```python
from build123d import *

# Parameters (mm, degrees)
SKETCH_1_W          = 35
SKETCH_1_H          = 25
EXTRUDE_1_DEPTH     = 10
SKETCH_1_4_W        = 10
SKETCH_1_4_H        = 25
EXTRUDE_2_DEPTH     = 15
SKETCH_2_W          = 10
SKETCH_2_H          = 13
CUT_EXTRUDE_1_DEPTH = 7
EXTRUDE_3_DEPTH     = 25
FILLET_1_R          = 5
CHAMFER_1_SIZE      = 1
SKETCH_5_R          = 1.5
EXTRUDE_4_DEPTH     = 5


with BuildPart() as part:
    # 草图1 → 凸台-拉伸1 (new body)
    with BuildSketch(Plane(origin=(0, 0, 0), x_dir=(1, 0, 0), z_dir=(0, 1, 0))):
        with Locations((5, 0)):
            Rectangle(SKETCH_1_W, SKETCH_1_H)
    extrude(amount=EXTRUDE_1_DEPTH)

    # 草图1<4> → 凸台-拉伸2 (add)
    with BuildSketch(Plane(origin=(0, 0, 0), x_dir=(1, 0, 0), z_dir=(0, 1, 0))):
        with Locations((-17.5, 0)):
            Rectangle(SKETCH_1_4_W, SKETCH_1_4_H)
    extrude(amount=EXTRUDE_2_DEPTH)

    # 草图2 → 切除-拉伸1 (cut)
    with BuildSketch(Plane.ZY.offset(22.5)):
        with Locations((5, 7.5)):
            Rectangle(SKETCH_2_W, SKETCH_2_H)
        with Locations((-5, 7.5)):
            Rectangle(SKETCH_2_W, SKETCH_2_H)
    extrude(amount=-CUT_EXTRUDE_1_DEPTH, mode=Mode.SUBTRACT)

    # 草图3 → 凸台-拉伸3 (add, through all)
    with BuildSketch(Plane.XY.offset(12.5)):
        Polygon((-7.5, 10), (-12.5, 15), (-12.5, 12.5), (-12.5, 10), (-10, 10), align=None)
    extrude(amount=-EXTRUDE_3_DEPTH)

    # 圆角1
    fillet_1_edges = [part.edges().sort_by_distance(p)[0] for p in [
        (-12.5, 15, 0),
    ]]
    fillet(fillet_1_edges, radius=FILLET_1_R)

    # 倒角1
    chamfer_1_edges = [part.edges().sort_by_distance(p)[0] for p in [
        (-18.535533906, 15, -12.5),
        (-22.5, 0, 0),
        (-22.5, 7.5, -12.5),
        (-22.5, 7.5, 12.5),
        (-22.5, 15, 0),
        (-18.535533906, 15, 12.5),
        (22.5, 10, 0),
        (7.5, 10, -12.5),
        (7.5, 10, 12.5),
        (-9.267766953, 11.767766953, 12.5),
        (-9.267766953, 11.767766953, -12.5),
        (22.5, 0, 0),
        (-12.65765065, 14.619397663, 12.5),
        (-12.65765065, 14.619397663, -12.5),
        (0, 0, 12.5),
        (0, 0, -12.5),
        (22.5, 5, -12.5),
        (22.5, 5, 12.5),
    ]]
    chamfer(chamfer_1_edges, length=CHAMFER_1_SIZE - 0.0001)  # a hair under: the kernel refuses the full size

    # 草图5 → 凸台-拉伸4 (add)
    with BuildSketch(Plane(origin=(22.5, 0, 0), x_dir=(0, 0, -1), z_dir=(1, 0, 0))):
        with Locations((-7.5, 5)):
            Circle(SKETCH_5_R)
        with Locations((7.5, 5)):
            Circle(SKETCH_5_R)
    extrude(amount=EXTRUDE_4_DEPTH)


solid = part.part
```
Could you check a few things on this model? Use its own coordinates, in mm. A direction names the side the tool comes from. Round coordinates to 2 decimals unless told otherwise and drop trailing zeros. Loops run counter-clockwise (first coordinate to the right, second up) from the corner with the lowest first, then second, coordinate; pieces in that order, holes last. Notation, with made-up numbers: M 65.25,3.5 L 124.25,3.5 A23 cw 124.25,36.5 Z; hole C 87,33.25 d11. An arc over 180 degrees is marked long. Write item = value, one per line.
1. I want a section at D-D, the plane x = 0. Write out the boundary of the cut face in (y, z).
Results below:
outline = M 0,-11.5 L 1,-12.5 L 9,-12.5 L 10,-11.5 L 10,11.5 L 9,12.5 L 1,12.5 L 0,11.5 Z
2. Will these pins go through, and if not, where does the flat tip stop? P1, Ø4, axis at x = -3, z = 3, coming from the +Y side; P2, Ø1, axis at y = 7, z = -1.5, coming from the -X side; P3, Ø2, axis at y = 1.5, z = 2, coming from the +X side; P4, Ø6, axis at x = 22, y = 7.5, coming from the -Z side.
Results below:
P1 = 10
P2 = -15.5
P3 = 22.5
P4 = -12.5
3. Thinking about a two-plate mould opening in Z: for faces 1 (the face through (21.8, 0.7, -11.9)), 2 (the face through (25, 4.1, -6.3)), 3 (the face through (-21.8, 14.4, 11.8)), which applies, +Z half, -Z half, draft (parallel to the pull), parting line (faces both ways), or undercut?
Results below:
face_1 = -Z half
face_2 = undercut
face_3 = +Z half
4. Which directions (+Z, -Z, +X, -X, +Y, -Y) give clear straight access to the entire face, cutting with the end or side of a thin tool? Please do faces 4 (the face through (6.6, 9.5, 12)), 5 (the face through (-19, 1, 0)), 6 (the face through (7, 10, 0)).
Results below:
face_4 = +Z, +X, +Y
face_5 = -X
face_6 = +Z, -Z, +X, +Y
5. I want a section at A-A, the plane y = 5. Write out the boundary of the cut face in (x, z), and give its area (3 significant figures).
Results below:
outline = M -22.5,-11.5 L -21.5,-12.5 L 21.5,-12.5 L 22.5,-11.5 L 22.5,-9 L 27.5,-9 L 27.5,-6 L 22.5,-6 L 22.5,6 L 27.5,6 L 27.5,9 L 22.5,9 L 22.5,11.5 L 21.5,12.5 L -21.5,12.5 L -22.5,11.5 L -22.5,10 L -15.5,10 L -15.5,-10 L -22.5,-10 Z
area = 1,010 mm²
6. I want a section at C-C, the plane x = -17. Write out the boundary of the cut face in (y, z), and give its area (3 significant figures).
Results below:
outline = M 0,-11.5 L 1,-12.5 L 14,-12.5 L 15,-11.5 L 15,11.5 L 14,12.5 L 1,12.5 L 0,11.5 Z; hole M 1,-10 L 14,-10 L 14,10 L 1,10 Z
area = 113 mm²
7. I need wall thicknesses on probe 1 along Y at (x, z) = (-17.5, -4.75); probe 2 along X at (y, z) = (8.5, 8.5); probe 3 along Y at (x, z) = (3, 3.75). Which ranges of each line are inside material? Lowest first, please.
Results below:
probe_1 = 0 to 1, 14 to 15
probe_2 = -15.5 to 22.5
probe_3 = 0 to 10
